```python
from build123d import *

# Parameters (mm, degrees)
F0_W     = 48.26
F0_H     = 31.75
F1_DEPTH = 12.7
F2_W     = 48.26
F2_H     = 25.781
F3_DEPTH = 4.7625
F5_DEPTH = 28.575
F6_R     = 3.2639
F7_DEPTH = 7.9375
F6_R_2   = 8.89
F8_DEPTH = 2.54
F9_R     = 1.5875
F10_R    = 1.5875
F11_R    = 1.5875
F12_R    = 1.5875


with BuildPart() as f1:
    # F0 (on Top) → F1 (new body)
    with BuildSketch(Plane.XY):
        Rectangle(F0_W, F0_H)
    extrude(amount=F1_DEPTH)

    # F2 (on face) → F3 (cut)
    with BuildSketch(Plane.XY.offset(12.7)):
        Rectangle(F2_W, F2_H)
    extrude(amount=-F3_DEPTH, mode=Mode.SUBTRACT)

    # F4 (on face) → F5 (cut)
    with BuildSketch(Plane(origin=(0, 15.875, 0), x_dir=(-1, 0, 0), z_dir=(0, 1, 0))):
        with BuildLine():
            Line((-22.1851086635, 12.7), (-22.1851086635, 6.3481266276))
            ThreePointArc((-22.1851086635, 6.3481266276), (-19.0101086706, 3.1731266347), (-15.8351086777, 6.3481266276))
            Line((-15.8351086777, 6.3481266276), (-15.8351086777, 12.7))
            Line((-15.8351086777, 12.7), (-22.1851086635, 12.7))
        make_face()
        with BuildLine():
            Line((22.2424135567, 12.7), (15.9373691021, 12.7))
            Line((15.9373691021, 12.7), (15.9373691021, 6.3481266276))
            ThreePointArc((15.9373691021, 6.3481266276), (19.0898913294, 3.1956044003), (22.2424135567, 6.3481266276))
            Line((22.2424135567, 6.3481266276), (22.2424135567, 12.7))
        make_face()
    extrude(amount=-F5_DEPTH, mode=Mode.SUBTRACT)

    # F6 (on face) → F7 (cut, through all)
    with BuildSketch(Plane(origin=(0, 0, 0), x_dir=(1, 0, 0), z_dir=(0, 0, -1))):
        Circle(F6_R)
    extrude(amount=-F7_DEPTH, mode=Mode.SUBTRACT)

    # F6 (on face) → F8 (cut)
    with BuildSketch(Plane(origin=(0, 0, 0), x_dir=(1, 0, 0), z_dir=(0, 0, -1))):
        Circle(F6_R_2)
        Circle(F6_R, mode=Mode.SUBTRACT)
    extrude(amount=-F8_DEPTH, mode=Mode.SUBTRACT)

    # F9
    f9_edges = [f1.edges().sort_by_distance(p)[0] for p in [
        (24.13, 0, 0),
        (0, 15.875, 0),
        (-24.13, 0, 0),
        (0, -15.875, 0),
        (-8.89, 0, 0),
    ]]
    fillet(f9_edges, radius=F9_R)

    # F10
    f10_edges = [f1.edges().sort_by_distance(p)[0] for p in [
        (-0.05113, 15.875, 12.7),
        (0, -15.875, 12.7),
    ]]
    fillet(f10_edges, radius=F10_R)

    # F11
    f11_edges = [f1.edges().sort_by_distance(p)[0] for p in [
        (-23.186207, 15.875, 12.7),
    ]]
    fillet(f11_edges, radius=F11_R)

    # F12
    f12_edges = [f1.edges().sort_by_distance(p)[0] for p in [
        (23.157554, 15.875, 12.7),
    ]]
    fillet(f12_edges, radius=F12_R)


solid = f1.part
```
Can you work these out from the model? Positions are in its coordinate system, mm. A direction names the side the tool comes from. Round coordinates to 2 decimals unless told otherwise and drop trailing zeros. Loops run counter-clockwise (first coordinate to the right, second up) from the corner with the lowest first, then second, coordinate; pieces in that order, holes last. Notation, with made-up numbers: (-29.5, 29.25) -> (-20.5, 29.25) arc R8 ccw to (-20.5, 41.25) -> close; hole circle Ø1 at (58, -17.5). An arc over 180 degrees is marked (long way). One line per item, written item: value. Start each with the question number.
1. If we section it at C-C, the plane x = 0: Write out the boundary of the cut face in (y, z) (1 decimal), then the cut area to 3 significant figures.
2. If we mould it in two halves opening along Y, with no side actions, what happens to faces 6 (the flat face through (0, -15.875, 6)), 7 (the flat face through (0, -12.89, 10)), 8 (the cylindrical face through (0.338, 15.398, 0.453)), 9 (the flat face through (23, 14, 12.7))? For each: pulls with the +Y half, pulls with the -Y half, needs draft (parallel to the pull), parting line crosses it, or undercut.
3. If I drill on probe 1 along X at (y, z) = (-8, 7.25); probe 2 along X at (y, z) = (0, 6.15); probe 3 along X at (y, z) = (14.5, 4), over which ranges is the centre line in solid material (lowest first)?
4. For pin 1 (7 mm diameter, centred on y = 4, z = 8.5, fed in from -X); pin 2 (3 mm diameter, centred on y = 2, z = 9.5, fed in from +X); pin 3 (8.5 mm diameter, centred on x = 0, y = 0, fed in from +Z); pin 4 (14 mm diameter, centred on x = 0, y = 0, fed in from -Z), each with a flat end and sliding along its axis, tell me the tip position at first contact or that it passes through.
5. For faces 1 (the flat face through (-15.937, 4, 7)), 2 (the cylindrical face through (-0.708, 3.186, 5.201)), 3 (the flat face through (0, 4, 2.54)), 4 (the flat face through (24.13, 0, 6)), 5 (the flat face through (-23, 12.89, 10)), which set-ups out of +Z, -Z, +X, -X, +Y, -Y let a thin tool reach every point of the face, with its end or its side?
6. If we section it at D-D, the plane x = 13: Write out the boundary of the cut face in (y, z) (1 decimal).
7. If we section it at A-A, the plane z = 9.5: Write out the boundary of the cut face in (x, y) (1 decimal).
Calculated:
1. outline: (-15.9, 1.6) arc R1.6 ccw to (-14.3, 0) -> (-10.5, 0) arc R1.6 ccw to (-8.9, 1.6) -> (-8.9, 2.5) -> (-3.3, 2.5) -> (-3.3, 7.9) -> (-12.9, 7.9) -> (-12.9, 12.7) -> (-14.3, 12.7) arc R1.6 ccw to (-15.9, 11.1) -> close; (3.3, 2.5) -> (8.9, 2.5) -> (8.9, 1.6) arc R1.6 ccw to (10.5, 0) -> (14.3, 0) arc R1.6 ccw to (15.9, 1.6) -> (15.9, 11.1) arc R1.6 ccw to (14.3, 12.7) -> (12.9, 12.7) -> (12.9, 7.9) -> (3.3, 7.9) -> close
1. area: 197 mm²
2. face 6: pulls with the -Y half
2. face 7: undercut
2. face 8: pulls with the +Y half
2. face 9: needs draft
3. probe 1: x = -24.13 to -22.24, -15.94 to 15.84, 22.19 to 24.13
3. probe 2: x = -24.13 to -22.24, -15.94 to -3.26, 3.26 to 15.84, 22.18 to 24.13
3. probe 3: x = -24.13 to -21.19, -16.99 to 16.87, 21.15 to 24.13
4. pin 1: stops at x = -24.13
4. pin 2: passes through
4. pin 3: stops at z = 7.94
4. pin 4: stops at z = 2.54
5. face 1: +Z, +Y
5. face 2: +Z, -Z
5. face 3: -Z
5. face 4: +Z, -Z, +X, +Y, -Y
5. face 5: +Z, +X, -X
6. outline: (-15.9, 1.6) arc R1.6 ccw to (-14.3, 0) -> (14.3, 0) arc R1.6 ccw to (15.9, 1.6) -> (15.9, 11.1) arc R1.6 ccw to (14.3, 12.7) -> (12.9, 12.7) -> (12.9, 7.9) -> (-12.9, 7.9) -> (-12.9, 12.7) -> (-14.3, 12.7) arc R1.6 ccw to (-15.9, 11.1) -> close
7. outline: (-24.1, -15.9) -> (24.1, -15.9) -> (24.1, -12.9) -> (-24.1, -12.9) -> close; (-24.1, 12.9) -> (-22.2, 12.9) -> (-22.2, 15.9) -> (-24.1, 15.9) -> close; (-15.9, 12.9) -> (15.8, 12.9) -> (15.8, 15.9) -> (-15.9, 15.9) -> close; (22.2, 12.9) -> (24.1, 12.9) -> (24.1, 15.9) -> (22.2, 15.9) -> close
